For this review, use the dimensioned drawing (mm, ordinates from the lowest corner) and the shaded views. Coordinates: 2 decimals unless noted, no trailing zeros. Order: outer loops, then holes, each group sorted by start corner. A loop starts at its lowest first (then second) coordinate and runs counter-clockwise, first axis right, second up. Notation, with made-up numbers: (56, 89) -> (114, 89) arc R17 cw to (114, 121) -> close; hole circle Ø7 at (29.25, 54.5). An arc over 180 degrees is marked (long way). Use CSV: the item, a comma, the result in double quotes. Start each with the question number.
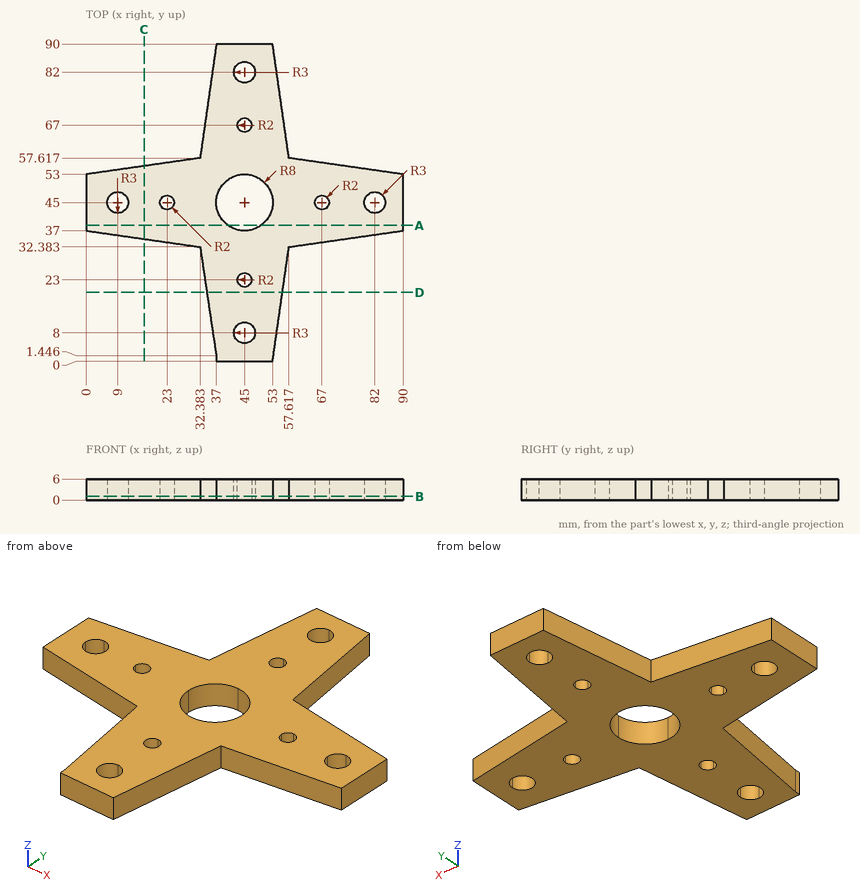
Q1. Add section C-C, the plane x = 16.5. State the section outline as (y, z) points.
Q2. Add section D-D, the plane y = 19.5. State the section outline as (x, z) points.
Q3. Add section A-A, the plane y = 38.5. State the section outline as (x, z) points.
Q4. To check wall thickness, follow probe 1 along Y at (x, z) = (50, 2.9) (1 decimal); probe 2 along Y at (x, z) = (9, 1.1); probe 3 along X at (y, z) = (31, 0.3). State the ranges of each line that lie inside material, in increasing order.
Q5. Clearance check with flat-ended pins moving along their axes: pin 1 Ø3 at (y, z) = (65, 4) entering from -X; pin 2 Ø1.2 at (y, z) = (0.5, 3.5) entering from -X. State where each tip first meets the part, or that it passes through.
Q6. Add section B-B, the plane z = 1.1. State how many separate pieces and enclosed holes the cut face has, then the cut area to 3 significant figures.
Answer block:
1,outline,"(34.65, 0) -> (55.35, 0) -> (55.35, 6) -> (34.65, 6) -> close"
2,outline,"(34.31, 0) -> (55.78, 0) -> (55.78, 6) -> (34.31, 6) -> close"
3,outline,"(0, 0) -> (40.34, 0) -> (40.34, 6) -> (0, 6) -> close; (49.66, 0) -> (90, 0) -> (90, 6) -> (49.66, 6) -> close"
4,probe 1,"y = 0 to 38.8, 51.2 to 90"
4,probe 2,"y = 35.72 to 42, 48 to 54.28"
4,probe 3,"x = 32.59 to 57.42"
5,pin 1,"stops at x = 33.22"
5,pin 2,"stops at x = 37"
6,separate pieces,"1"
6,enclosed holes,"9"
6,area,"2,940 mm²"
